from build123d import *

# Parameters (mm, degrees)
F0_R     = 9.349466
F1_DEPTH = 50.8
F0_W     = 93.26841
F0_H     = 57.62465
F2_DEPTH = 25.4
F4_DEPTH = 25.4
F5_DEPTH = 76.2


with BuildPart() as f1:
    # F0 (on Top) → F1 (new body)
    with BuildSketch(Plane.XY):
        Circle(F0_R)
    extrude(amount=F1_DEPTH)

    # F0 (on Top) → F2 (join)
    with BuildSketch(Plane.XY):
        Rectangle(F0_W, F0_H)
        Circle(F0_R, mode=Mode.SUBTRACT)
    extrude(amount=F2_DEPTH)

    # F3 (on Front) → F4 (cut)
    with BuildSketch(Plane.XZ):
        Polygon((29.052887, 52.606806), (-13.472474, 52.606806), (29.052887, 30.427627), align=None)
    extrude(amount=-F4_DEPTH, mode=Mode.SUBTRACT)

    # F3 (on Front) → F5 (cut)
    with BuildSketch(Plane.XZ):
        Polygon((29.052887, 52.606806), (-13.472474, 52.606806), (29.052887, 30.427627), align=None)
    extrude(amount=F5_DEPTH, mode=Mode.SUBTRACT)


solid = f1.part
Geometry: final body of the model. Coordinates: model frame, mm. A direction names the side the tool comes from. Round coordinates to 2 decimals unless told otherwise and drop trailing zeros. Loops run counter-clockwise (first coordinate to the right, second up) from the corner with the lowest first, then second, coordinate; pieces in that order, holes last.
Q1. Section D-D on y = -13. Return loops of the section in (x, z), plus the area to 3 significant figures.
Q2. Access query for faces 1 (the flat face through (-1, 0, 0)), 2 (the cylindrical face through (-9.34, 0.41, 34.97)). Directions: +Z, -Z, +X, -X, +Y, -Y. A direction counts if a zero-diameter tool reaches every point of the face in a straight line with its end or side. Return the directions, or none.
Q3. Section A-A on y = 0. Return loops of the section in (x, z), plus the area to 3 significant figures.
Q4. Section B-B on z = 31. Return loops of the section in (x, y).
Q5. Section C-C on x = -4.5. Return loops of the section in (y, z), plus the area to 3 significant figures.
Q6. Pin query (flat end, axial travel): P1, Ø8, axis at x = -33.5, y = 1, coming from the +Z side; P2, Ø4, axis at y = 3.5, z = 37, coming from the -X side. Return the tip coordinate at first contact, or that it passes through.
Q7. Material intervals for L1, parallel to Z at x = 25, y = -16; L2, parallel to Y at x = -0.5, z = 27.5; L3, parallel to X at y = 7, z = 48, sorted ascending.
Evaluation:
1. outline: (-46.63, 0) - (46.63, 0) - (46.63, 25.4) - (-46.63, 25.4) - close
1. area: 2,370 mm2
2. face 1: -Z, +X, -X, +Y, -Y
2. face 2: +Z
3. outline: (-46.63, 0) - (46.63, 0) - (46.63, 25.4) - (9.35, 25.4) - (9.35, 40.7) - (-9.35, 50.46) - (-9.35, 25.4) - (-46.63, 25.4) - close
3. area: 2,750 mm2
4. outline: circle Ø18.7 at (0, 0)
5. outline: (-28.81, 0) - (28.81, 0) - (28.81, 25.4) - (8.2, 25.4) - (8.2, 47.93) - (-8.2, 47.93) - (-8.2, 25.4) - (-28.81, 25.4) - close
5. area: 1,830 mm2
6. P1: stops at z = 25.4
6. P2: stops at x = -9.23
7. L1: z = 0 to 25.4
7. L2: y = -9.34 to 9.34
7. L3: x = -6.2 to -4.64
